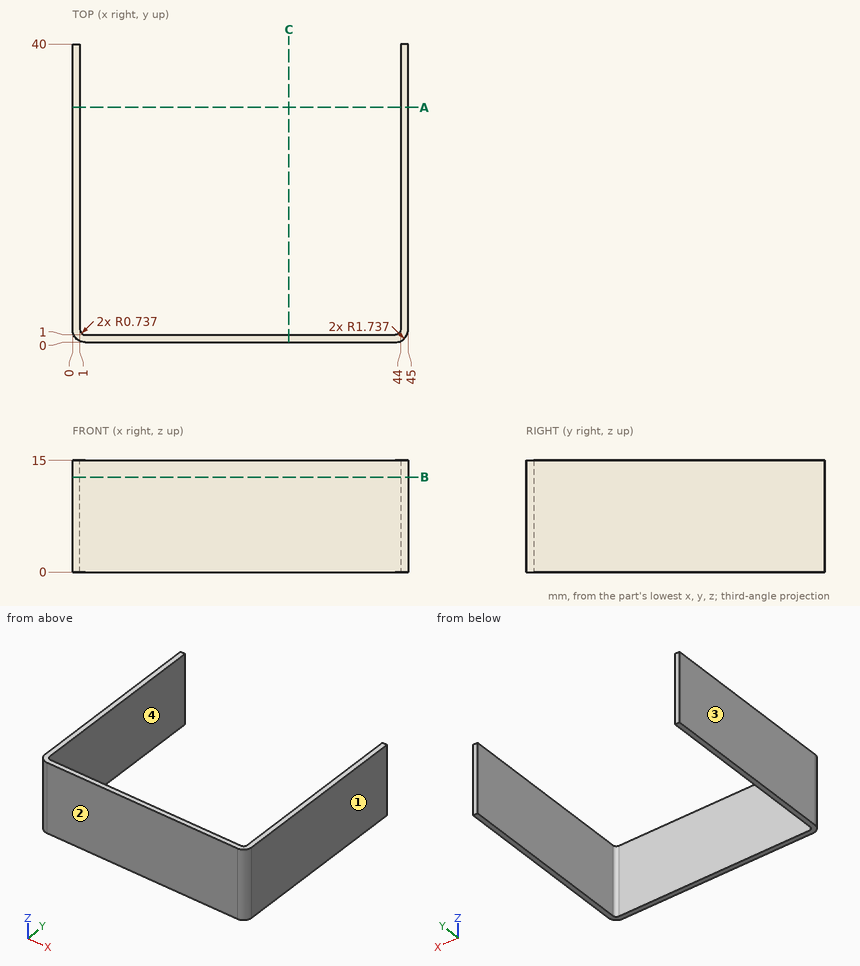
Part print with two shaded views. Sizes in mm from the minimum x, y, z corner. Coordinates: 2 decimals unless noted, no trailing zeros. Write each loop counter-clockwise with the first axis right and the second up, starting at its lowest first coordinate (ties: lowest second). Pieces come first, ordered by that corner, then holes.
(1) Cut at C-C on x = 29. List the corners of the cut face in (y, z).
(2) Mould opens along X. For the marked faces 1, 2, 3 and 4 say: pulls with the +X half, pulls with the -X half, needs draft (parallel to the pull), parting line crosses it, or undercut.
(3) Pin check, flat tip, straight feed: pin 1 Ø7.5 at (x, z) = (24.5, 9.5) entering from +Y. Stop position of the tip, or through.
(4) Cut at B-B on z = 12.75. List the corners of the cut face in (x, y).
(5) Drill centre lines: line 1 (X direction, y = 16.5, z = 2); line 2 (Y direction, x = 10, z = 7.25). Where is each one in solid material? Low to high.
(6) Cut at A-A on y = 31.5. List the corners of the cut face in (x, z).
Working result:
1. outline: (0, 0) - (1, 0) - (1, 15) - (0, 15) - close
2. face 1: pulls with the +X half
2. face 2: needs draft
2. face 3: pulls with the -X half
2. face 4: undercut
3. pin 1: stops at y = 1
4. outline: (0, 1.74) arc R1.74 ccw to (1.74, 0) - (43.26, 0) arc R1.74 ccw to (45, 1.74) - (45, 40) - (44, 40) - (44, 1.74) arc R0.74 cw to (43.26, 1) - (1.74, 1) arc R0.74 cw to (1, 1.74) - (1, 40) - (0, 40) - close
5. line 1: x = 0 to 1, 44 to 45
5. line 2: y = 0 to 1
6. outline: (0, 0) - (1, 0) - (1, 15) - (0, 15) - close; (44, 0) - (45, 0) - (45, 15) - (44, 15) - close
